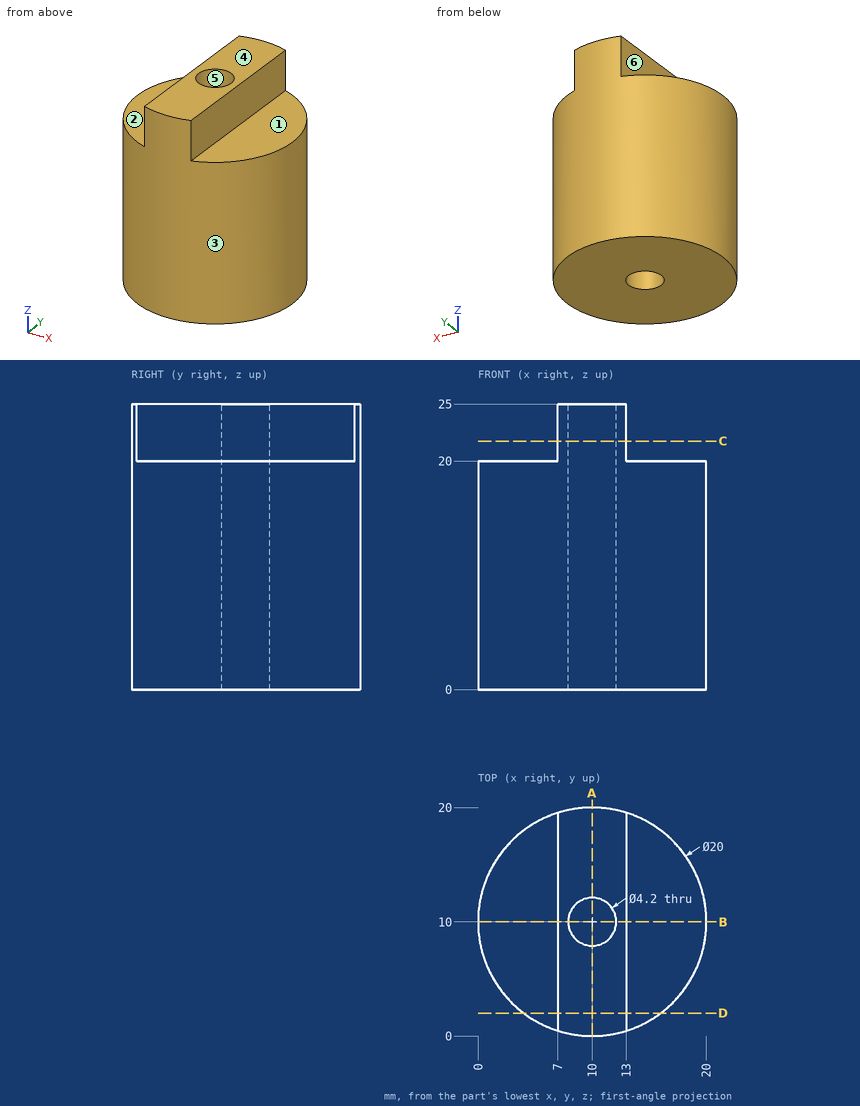
Job drawing, mm, ordinate dimensions from the low corner. One solid piece. A direction names the side the tool comes from. Round coordinates to 2 decimals unless told otherwise and drop trailing zeros. Write each loop counter-clockwise with the first axis right and the second up, starting at its lowest first coordinate (ties: lowest second). Pieces come first, ordered by that corner, then holes. Notation, with made-up numbers: M 16.25,79 L 43.25,79 A34 ccw 43.25,109 Z; hole C 31,50 d2. An arc over 180 degrees is marked long. Return JSON: item names as keys, results as strings. Group by question number.
(1) Saw through at D-D on y = 2. Write the cut outline in (x, z), then the cut area to 3 significant figures.
(2) Drill centre lines: probe 1 along Y at (x, z) = (10, 9.5); probe 2 along Z at (x, y) = (16.5, 6.75). Where is each one in solid material? Low to high.
(3) Saw through at B-B on y = 10. Write the cut outline in (x, z), then the cut area to 3 significant figures.
(4) Saw through at C-C on z = 21.75. Write the cut outline in (x, y), then the cut area to 3 significant figures.
(5) Two-plate mould, pull along X, no slides. Class the marked faces 4, 5 and 6: +X half, -X half, draft (parallel to the pull), parting line (faces both ways), or undercut.
(6) Pin check, flat tips, straight feed: pin 1 Ø7.5 at (x, y) = (3.5, 14.5) entering from +Z; pin 2 Ø2.5 at (y, z) = (14, 23.5) entering from -X; pin 3 Ø2.5 at (y, z) = (6, 22) entering from +X; pin 4 Ø4 at (x, y) = (3, 4.5) entering from +Z. Stop position of each tip, or through.
(7) Which spindle directions (+Z, -Z, +X, -X, +Y, -Y) get a long thin tool onto all of the face, cutting with end or side? Do the marked faces 1, 2 and 3. Say none if no direction does.
(8) Saw through at A-A on x = 10. Write the cut outline in (y, z).
Returned:
{
 "1": {"outline": "M 4,0 L 16,0 L 16,20 L 13,20 L 13,25 L 7,25 L 7,20 L 4,20 Z", "area": "270 mm²"},
 "2": {"probe 1": "0 to 7.9, 12.1 to 20", "probe 2": "0 to 20"},
 "3": {"outline": "M 0,0 L 7.9,0 L 7.9,25 L 7,25 L 7,20 L 0,20 Z; M 12.1,0 L 20,0 L 20,20 L 13,20 L 13,25 L 12.1,25 Z", "area": "325 mm²"},
 "4": {"outline": "M 7,0.46 A10 ccw 13,0.46 L 13,19.54 A10 ccw 7,19.54 Z; hole C 10,10 d4.2", "area": "104 mm²"},
 "5": {"face 4": "draft", "face 5": "undercut", "face 6": "-X half"},
 "6": {"pin 1": "z = 25", "pin 2": "x = 7", "pin 3": "x = 13", "pin 4": "z = 20"},
 "7": {"face 1": "+Z, +X, +Y, -Y", "face 2": "+Z, -X, +Y, -Y", "face 3": "+Z, -Z"},
 "8": {"outline": "M 0,0 L 7.9,0 L 7.9,25 L 0,25 Z; M 12.1,0 L 20,0 L 20,25 L 12.1,25 Z"}
}
